from build123d import *

# Parameters (mm, degrees)
BOX226_W          = 6
BOX226_H          = 4
BOX226_DEPTH      = 3
CYLINDER090_R     = 2
CYLINDER090_DEPTH = 5
CYLINDER089_R     = 2
CYLINDER089_DEPTH = 5
BOX223_W          = 6
BOX223_H          = 2.3
BOX223_DEPTH      = 28
FILLET056_R       = 2
BOX225_W          = 6
BOX225_H          = 4
BOX225_DEPTH      = 3
CYLINDER091_R     = 2
CYLINDER091_DEPTH = 5
BOX224_W          = 6
BOX224_H          = 3
BOX224_DEPTH      = 28


with BuildPart() as cube214:
    # Box226 → Box226 (new body)
    with BuildSketch(Plane(origin=(22.5, 53, -9.5), x_dir=(1, 0, 0), z_dir=(0, 0, 1))):
        with Locations((3, 2)):
            Rectangle(BOX226_W, BOX226_H)
    extrude(amount=BOX226_DEPTH)


with BuildPart() as cylinder171:
    # Cylinder090 → Cylinder090 (new body)
    with BuildSketch(Plane(origin=(25.5, 60, -27.5), x_dir=(1, 0, 0), z_dir=(0, -1, 0))):
        Circle(CYLINDER090_R)
    extrude(amount=CYLINDER090_DEPTH)


with BuildPart() as cylinder170:
    # Cylinder089 → Cylinder089 (new body)
    with BuildSketch(Plane(origin=(25.5, 60, -13.5), x_dir=(1, 0, 0), z_dir=(0, -1, 0))):
        Circle(CYLINDER089_R)
    extrude(amount=CYLINDER089_DEPTH)


with BuildPart() as fillet056:
    # Box223 → Box223 (new body)
    with BuildSketch(Plane(origin=(22.5, 57, -34.5), x_dir=(1, 0, 0), z_dir=(0, 0, 1))):
        with Locations((3, 1.15)):
            Rectangle(BOX223_W, BOX223_H)
    extrude(amount=BOX223_DEPTH)

    # Cut113: cut Cylinder170
    add(cylinder170.part, mode=Mode.SUBTRACT)

    # Cut114: cut Cylinder171
    add(cylinder171.part, mode=Mode.SUBTRACT)

    # Fillet056
    fillet056_edges = [fillet056.edges().sort_by_distance(p)[0] for p in [
        (25.5, 59.3, -6.5),
        (25.5, 59.3, -34.5),
    ]]
    fillet(fillet056_edges, radius=FILLET056_R)


with BuildPart() as cube213:
    # Box225 → Box225 (new body)
    with BuildSketch(Plane(origin=(22.5, 53, -34.5), x_dir=(1, 0, 0), z_dir=(0, 0, 1))):
        with Locations((3, 2)):
            Rectangle(BOX225_W, BOX225_H)
    extrude(amount=BOX225_DEPTH)


with BuildPart() as cylinder172:
    # Cylinder091 → Cylinder091 (new body)
    with BuildSketch(Plane(origin=(25.5, 54, -20.5), x_dir=(1, 0, 0), z_dir=(0, -1, 0))):
        Circle(CYLINDER091_R)
    extrude(amount=CYLINDER091_DEPTH)


with BuildPart() as fusion071:
    # Box224 → Box224 (new body)
    with BuildSketch(Plane(origin=(22.5, 50, -34.5), x_dir=(1, 0, 0), z_dir=(0, 0, 1))):
        with Locations((3, 1.5)):
            Rectangle(BOX224_W, BOX224_H)
    extrude(amount=BOX224_DEPTH)

    # Cut115: cut Cylinder172
    add(cylinder172.part, mode=Mode.SUBTRACT)

    # Fusion071: union Cube214, Fillet056, Cube213
    add(cube214.part)
    add(fillet056.part)
    add(cube213.part)


solid = fusion071.part
The listing builds one solid part. Answer for the finished solid, in the listing's coordinates (mm). A direction names the side the tool comes from. Coordinates: 2 decimals unless noted, no trailing zeros. Write each loop counter-clockwise with the first axis right and the second up, starting at its lowest first coordinate (ties: lowest second). Pieces come first, ordered by that corner, then holes. Notation, with made-up numbers: (-3.75, 39) - (21.25, 39) arc R13 ccw to (21.25, 55) - close; hole circle Ø5 at (-35.75, 48). An arc over 180 degrees is marked (long way). Put each result on its own line as item: value.
1. The part is cut by section B-B on y = 56. Give the vertices of the cut face in (x, z), plus the area to 3 significant figures.
Answer sheet:
outline: (22.5, -34.5) - (28.5, -34.5) - (28.5, -31.5) - (22.5, -31.5) - close; (22.5, -9.5) - (28.5, -9.5) - (28.5, -6.5) - (22.5, -6.5) - close
area: 36.0 mm^2
2. A tool of negligible diameter and unlimited length cuts with its end or side. For faces 1 (the face through (25, 55, -9.5)), 2 (the face through (24.026, 51.521, -19.148)), 3 (the face through (25, 54, -6.5)), 4 (the face through (24.026, 58.166, -12.148)), 5 (the face through (28.5, 52.5, -20.7)), from which of +Z, -Z, +X, -X, +Y, -Y can it reach the whole face along a straight path? Write none if from no direction.
Answer sheet:
face 1: +X, -X
face 2: -Y
face 3: +Z, +X, -X, +Y, -Y
face 4: +Y
face 5: +Z, -Z, +X, +Y, -Y
3. Determine the mould class of faces 6 (the face through (25, 55, -31.5)), 7 (the face through (25.54, 58.73, -7.1)), 8 (the face through (23, 53, -21)), 9 (the face through (22.5, 52.5, -20.7)) for opening direction Z: pulls with the +Z half, pulls with the -Z half, needs draft (parallel to the pull), parting line crosses it, or undercut.
Answer sheet:
face 6: undercut
face 7: pulls with the +Z half
face 8: undercut
face 9: needs draft
4. Find the intervals of material crossed by line 1 along Y through (x, z) = (27.8, -30.75); line 2 along Z through (x, y) = (25.5, 51.7); line 3 along X through (y, z) = (57.7, -27.5), in increasing order. Write a range as from..to.
Answer sheet:
line 1: y = 50..53, 57..59.3
line 2: z = -34.5..-22.5, -18.5..-6.5
line 3: x = 22.5..23.5, 27.5..28.5
5. The part is cut by section D-D on z = -31. Give the vertices of the cut face in (x, y), plus the area to 3 significant figures.
Answer sheet:
outline: (22.5, 50) - (28.5, 50) - (28.5, 53) - (22.5, 53) - close; (22.5, 57) - (28.5, 57) - (28.5, 59.3) - (22.5, 59.3) - close
area: 31.8 mm^2
6. The part is cut by section A-A on z = -13.5. Give the vertices of the cut face in (x, y), plus the area to 3 significant figures.
Answer sheet:
outline: (22.5, 50) - (28.5, 50) - (28.5, 53) - (22.5, 53) - close; (22.5, 57) - (23.5, 57) - (23.5, 59.3) - (22.5, 59.3) - close; (27.5, 57) - (28.5, 57) - (28.5, 59.3) - (27.5, 59.3) - close
area: 22.6 mm^2
7. The part is cut by section C-C on x = 27.9. Give the vertices of the cut face in (y, z), plus the area to 3 significant figures.
Answer sheet:
outline: (50, -34.5) - (57.3, -34.5) arc R2 ccw to (59.3, -32.5) - (59.3, -8.5) arc R2 ccw to (57.3, -6.5) - (50, -6.5) - close; hole (53, -31.5) - (57, -31.5) - (57, -9.5) - (53, -9.5) - close
area: 171 mm^2
